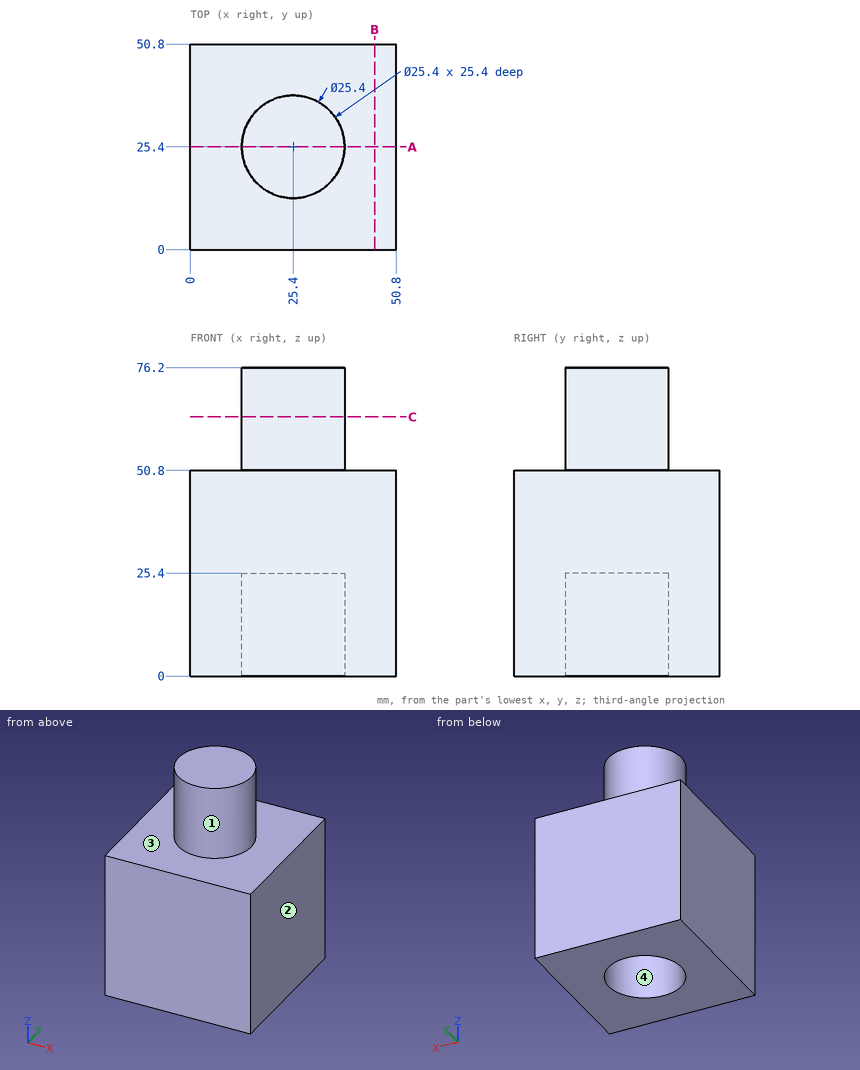
Geometry check sheet. Reference: drawing and pictorial views, mm from the part's lowest x, y, z. Give positions to 0.01 mm unless a question says otherwise; leave off trailing zeros. Order: outer loops, then holes, each group sorted by start corner. A loop starts at its lowest first (then second) coordinate and runs counter-clockwise, first axis right, second up. Notation, with made-up numbers: M -12,-39.75 L 0,-39.75 A16 ccw 0,-12.75 Z; hole C 14.25,51.5 d10. An arc over 180 degrees is marked long. Answer in a Markdown table with one row per item.
1) Thickness scan on L1, parallel to Y at x = 25.4, z = 14.25; L2, parallel to X at y = 25, z = 5; L3, parallel to Z at x = 17.5, y = 42.5. Record the ranges inside material, lowest first. Write a range as [from, to].
Filled sheet:
| item | result |
|---|---|
| L1 | y = [0, 12.7], [38.1, 50.8] |
| L2 | x = [0, 12.71], [38.09, 50.8] |
| L3 | z = [0, 50.8] |
2) Cross-section at C-C, the plane z = 64. Enter the section's corners in (x, y).
Filled sheet:
| item | result |
|---|---|
| outline | C 25.4,25.4 d25.4 |
3) Release check for a two-part mould opening along X. For the marked faces 1, 2, 3 and 4 record: +X half, -X half, draft (parallel to the pull), parting line (faces both ways), or undercut.
Filled sheet:
| item | result |
|---|---|
| face 1 | parting line |
| face 2 | +X half |
| face 3 | draft |
| face 4 | undercut |
4) Cross-section at A-A, the plane y = 25.4. Enter the section's corners in (x, z).
Filled sheet:
| item | result |
|---|---|
| outline | M 0,0 L 12.7,0 L 12.7,25.4 L 38.1,25.4 L 38.1,0 L 50.8,0 L 50.8,50.8 L 38.1,50.8 L 38.1,76.2 L 12.7,76.2 L 12.7,50.8 L 0,50.8 Z |
5) Gauge pin test, flat ends, axial feed: P1, Ø3, axis at y = 18, z = 52.5, coming from the +X side; P2, Ø5, axis at x = 36, y = 36, coming from the +Z side; P3, Ø10, axis at y = 37.5, z = 62, coming from the +X side. Record the tip position at first contact, or that the pin passes through.
Filled sheet:
| item | result |
|---|---|
| P1 | stops at x = 36.65 |
| P2 | stops at z = 76.2 |
| P3 | stops at x = 35.93 |
6) Cross-section at B-B, the plane x = 45.5. Enter the section's corners in (y, z).
Filled sheet:
| item | result |
|---|---|
| outline | M 0,0 L 50.8,0 L 50.8,50.8 L 0,50.8 Z |
